```python
from build123d import *

# Parameters (mm, degrees)
IZIM1_W                     = 50
IZIM1_H                     = 75
Y_KSEKLIK_EKSTR_ZYON1_DEPTH = 15
IZIM2_W                     = 50
IZIM2_H                     = 15
Y_KSEKLIK_EKSTR_ZYON2_DEPTH = 50
Y_KSEKLIK_EKSTR_ZYON3_DEPTH = 5
IZIM5_W                     = 10
IZIM5_H                     = 8
KES_EKSTR_ZYON1_DEPTH       = 76
IZIM6_W                     = 10
IZIM6_H                     = 8
KES_EKSTR_ZYON2_DEPTH       = 51


with BuildPart() as part:
    # Çizim1 → Yükseklik-Ekstrüzyon1 (new body)
    with BuildSketch(Plane(origin=(0, 0, 0), x_dir=(1, 0, 0), z_dir=(0, 1, 0))):
        Rectangle(IZIM1_W, IZIM1_H)
    extrude(amount=Y_KSEKLIK_EKSTR_ZYON1_DEPTH)

    # Çizim2 → Yükseklik-Ekstrüzyon2 (add)
    with BuildSketch(Plane(origin=(0, 15, 0), x_dir=(1, 0, 0), z_dir=(0, 1, 0))):
        with Locations((0, 30)):
            Rectangle(IZIM2_W, IZIM2_H)
    extrude(amount=Y_KSEKLIK_EKSTR_ZYON2_DEPTH)

    # Çizim4 → Yükseklik-Ekstrüzyon3 (add, symmetric)
    with BuildSketch(Plane(origin=(0, 0, 0), x_dir=(0, 0, -1), z_dir=(1, 0, 0))):
        Polygon((22.5, 65), (-37.5, 15), (22.5, 15), align=None)
    extrude(amount=Y_KSEKLIK_EKSTR_ZYON3_DEPTH, both=True)

    # Çizim5 → Kes-Ekstrüzyon1 (cut, through all)
    with BuildSketch(Plane.XY.offset(37.5)):
        with Locations((0, 4)):
            Rectangle(IZIM5_W, IZIM5_H)
    extrude(amount=-KES_EKSTR_ZYON1_DEPTH, mode=Mode.SUBTRACT)

    # Çizim6 → Kes-Ekstrüzyon2 (cut, through all)
    with BuildSketch(Plane(origin=(25, 0, 0), x_dir=(0, 0, -1), z_dir=(1, 0, 0))):
        with Locations((0, 4)):
            Rectangle(IZIM6_W, IZIM6_H)
    extrude(amount=-KES_EKSTR_ZYON2_DEPTH, mode=Mode.SUBTRACT)


solid = part.part
```
Geometry check sheet. Reference: the model listing, model coordinates, mm. A direction names the side the tool comes from. Coordinates: 2 decimals unless noted, no trailing zeros. Order: outer loops, then holes, each group sorted by start corner. A loop starts at its lowest first (then second) coordinate and runs counter-clockwise, first axis right, second up. Notation, with made-up numbers: M 18,75 L 37,75 A12 ccw 37,87 Z; hole C 70,80 d5. An arc over 180 degrees is marked long. Answer as a JSON object with one key per item and string values.
Q1. Cross-section at B-B on z = -26.5. Record the cut outline in (x, y).
Results are:
{"outline": "M -25,0 L -5,0 L -5,8 L 5,8 L 5,0 L 25,0 L 25,65 L -25,65 Z"}
Q2. Tool access check on faces 5 (the flat face through (5, 29, -5)), 6 (the flat face through (15, 4, -5)), 7 (the flat face through (-15, 40, -22.5)). Record the directions out of +Z, -Z, +X, -X, +Y, -Y that give a thin tool (end or side, any length) a straight path to the whole face; none if there is none.
Results are:
{"face 5": "+Z, +X, +Y", "face 6": "+X, -X, -Y", "face 7": "+Z, -X, +Y"}
Q3. Cross-section at C-C on x = -10.5. Record the cut outline in (y, z).
Results are:
{"outline": "M 0,-37.5 L 65,-37.5 L 65,-22.5 L 15,-22.5 L 15,37.5 L 0,37.5 L 0,5 L 8,5 L 8,-5 L 0,-5 Z"}
Q4. Release check for a two-part mould opening along X. For faces 1 (the flat face through (5, 4, 21)), 2 (the flat face through (-25, 10, -16)), 3 (the flat face through (-5, 4, 21)), 4 (the flat face through (-15, 4, -5)) record: released by +X, released by -X, zero draft, split by the parting line, or undercut.
Results are:
{"face 1": "undercut", "face 2": "released by -X", "face 3": "undercut", "face 4": "zero draft"}
Q5. Depth check by flat-ended pin: pin 1 Ø2 at (y, z) = (44.5, -4.5) entering from -X; pin 2 Ø3 at (y, z) = (32, -15.5) entering from +X; pin 3 Ø4 at (x, z) = (7.5, 20) entering from +Y; pin 4 Ø25 at (y, z) = (52.5, 18) entering from +X. Enter the tip coordinate at first touch or a pass-through.
Results are:
{"pin 1": "stops at x = -5", "pin 2": "stops at x = 5", "pin 3": "stops at y = 15", "pin 4": "passes through"}
Q6. Cross-section at D-D on z = 18.5. Record the cut outline in (x, y).
Results are:
{"outline": "M -25,0 L -5,0 L -5,8 L 5,8 L 5,0 L 25,0 L 25,15 L 5,15 L 5,30.83 L -5,30.83 L -5,15 L -25,15 Z"}
Q7. Cross-section at A-A on y = 47.5. Record the cut outline in (x, z), and give its area (3 significant figures).
Results are:
{"outline": "M -25,-37.5 L 25,-37.5 L 25,-22.5 L 5,-22.5 L 5,-1.5 L -5,-1.5 L -5,-22.5 L -25,-22.5 Z", "area": "960 mm²"}
Q8. Scan lines: line 1 (X direction, y = 4, z = 22.5); line 2 (X direction, y = 35.5, z = -17); line 3 (Z direction, x = -21, y = 17). Record each from-to range of solid material in increasing order.
Results are:
{"line 1": "x = -25 to -5, 5 to 25", "line 2": "x = -5 to 5", "line 3": "z = -37.5 to -22.5"}
